from build123d import *

# Parameters (mm, degrees)
CROQUIS3_R            = 30
CORTAR_EXTRUIR1_DEPTH = 5
CROQUIS4_R            = 15
CORTAR_EXTRUIR2_DEPTH = 59.523499554
CROQUIS5_R            = 20
CORTAR_EXTRUIR3_DEPTH = 10


with BuildPart() as part:
    # Croquis2 → Revolución1 (revolve)
    with BuildSketch(Plane.XY, mode=Mode.PRIVATE) as revoluci_n1_sk:
        Polygon((0, 0), (30, 0), (40, -20), (0, -20), align=None)
    revolve(revoluci_n1_sk.sketch.rotate(Axis((0, 0, 0), (0, -1, 0)), 180), axis=Axis((0, 0, 0), (0, -1, 0)))

    # Croquis3 → Cortar-Extruir1 (cut)
    with BuildSketch(Plane(origin=(0, 0, 0), x_dir=(1, 0, 0), z_dir=(0, 1, 0))):
        with Locations(Location((0, 0, 0), (0, 0, 180))):
            Circle(CROQUIS3_R)
    extrude(amount=-CORTAR_EXTRUIR1_DEPTH, mode=Mode.SUBTRACT)

    # Croquis4 → Cortar-Extruir2 (cut, through all)
    with BuildSketch(Plane(origin=(0, -5, 0), x_dir=(1, 0, 0), z_dir=(0, 1, 0))):
        with Locations(Location((0, 0, 0), (0, 0, 180))):
            Circle(CROQUIS4_R)
    extrude(amount=-CORTAR_EXTRUIR2_DEPTH, mode=Mode.SUBTRACT)

    # Croquis5 → Cortar-Extruir3 (cut)
    with BuildSketch(Plane.XZ.offset(20)):
        Circle(CROQUIS5_R)
    extrude(amount=-CORTAR_EXTRUIR3_DEPTH, mode=Mode.SUBTRACT)


solid = part.part
Work out the finished part from the listing and answer in its coordinate system (mm). A direction names the side the tool comes from. Round coordinates to 2 decimals unless told otherwise and drop trailing zeros. Loops run counter-clockwise (first coordinate to the right, second up) from the corner with the lowest first, then second, coordinate; pieces in that order, holes last. Notation, with made-up numbers: (-37, 36.25) - (-23, 36.25) arc R20 ccw to (-23, 55.25) - close; hole circle Ø5 at (27.5, 46). An arc over 180 degrees is marked (long way). Use one line per item in the form item = value. Start each with the question number.
(1) Find section C-C on y = -16.5. Determine the outline of the cut face in (x, z).
(2) Which of the six approach directions +Z, -Z, +X, -X, +Y, -Y give full straight-line access (tool end or side, diameter ignored) to faces 1 (the face through (3, -10, 15)), 2 (the face through (-16.128, -2.465, 25.296)), 3 (the face through (9.4, -20, -18.3))?
(3) Find section D-D on y = -3.75. Determine the outline of the cut face in (x, z) (3 decimals), and give its area (3 significant figures).
(4) Flat-ended cylindrical pins translate along their axes: P1, Ø8, axis at y = -12, z = -9.5, coming from the +X side; P2, Ø10, axis at y = -15, z = -13, coming from the +X side; P3, Ø1.5, axis at x = 25, y = -10.5, coming from the -Z side. Find the tip coordinate at first contact, or state that the pin passes through.
(5) Find section A-A on x = 0. Determine the outline of the cut face in (y, z), and give its area (3 significant figures).
(6) Consider line 1 (Y direction, x = 0, z = 16.5); line 2 (Z direction, x = 11, y = -15.5); line 3 (Z direction, x = 26, y = -3.5). Determine where each line is inside the solid, lowest interval first.
(7) Find section B-B on z = 0. Determine the outline of the cut face in (x, y), and give its area (3 significant figures).
Answer list:
q1.outline = circle Ø76.5 at (0, 0); hole circle Ø40 at (0, 0)
q2.face_1 = -Y
q2.face_2 = +Y
q2.face_3 = +Z, -Z, +X, -X, -Y
q3.outline = circle Ø63.75 at (0, 0); hole circle Ø60 at (0, 0)
q3.area = 364 mm^2
q4.P1 = 37
q4.P2 = 38.25
q4.P3 = -25.75
q5.outline = (-20, -40) - (0, -30) - (-5, -30) - (-5, -15) - (-10, -15) - (-10, -20) - (-20, -20) - close; (-20, 20) - (-10, 20) - (-10, 15) - (-5, 15) - (-5, 30) - (0, 30) - (-20, 40) - close
q5.area = 550 mm^2
q6.line_1 = -10 to -5
q6.line_2 = -36.11 to -16.7, 16.7 to 36.11
q6.line_3 = -18.22 to -14.97, 14.97 to 18.22
q7.outline = (-40, -20) - (-20, -20) - (-20, -10) - (-15, -10) - (-15, -5) - (-30, -5) - (-30, 0) - close; (15, -10) - (20, -10) - (20, -20) - (40, -20) - (30, 0) - (30, -5) - (15, -5) - close
q7.area = 550 mm^2
